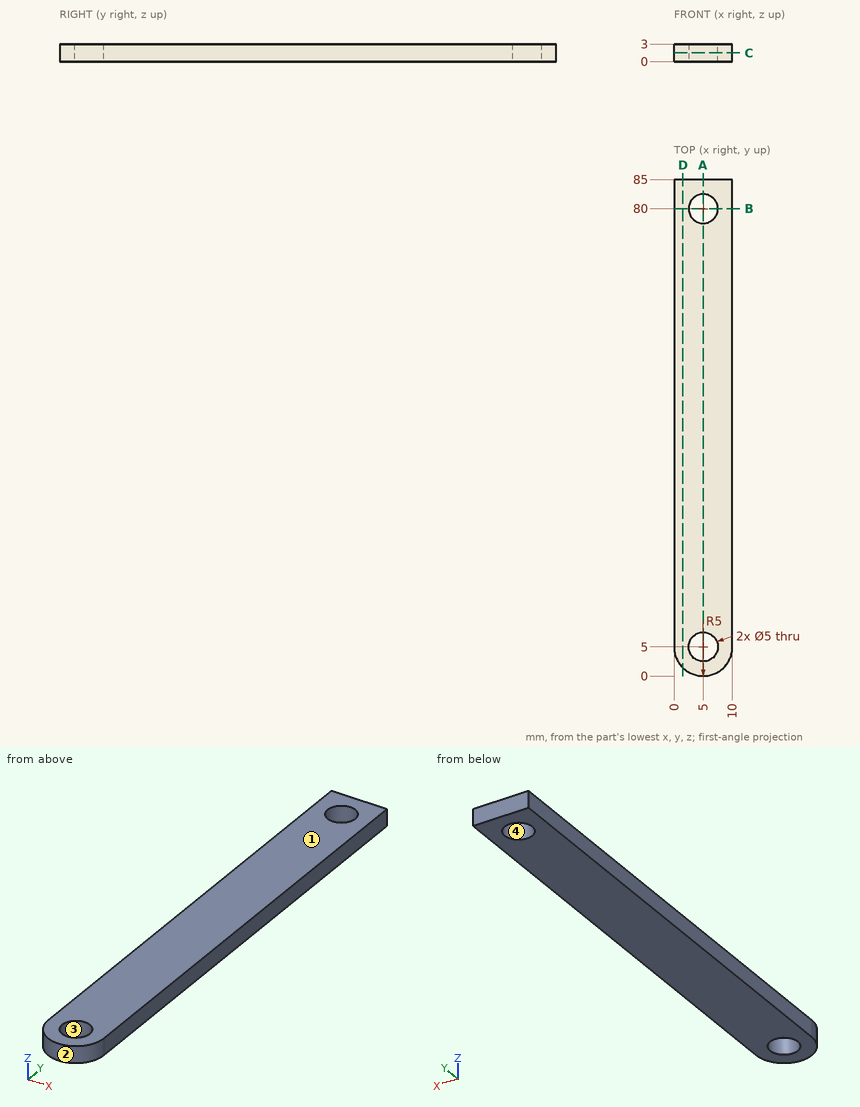
Here's the drawing with two shaded views (mm, measured from the low corner). I have some questions. Give positions to 0.01 mm unless a question says otherwise; leave off trailing zeros. Loops run counter-clockwise (first coordinate to the right, second up) from the corner with the lowest first, then second, coordinate; pieces in that order, holes last. Notation, with made-up numbers: (58.5, 62) - (99.5, 62) arc R12 cw to (99.5, 78) - close; hole circle Ø1 at (85, 56.25). An arc over 180 degrees is marked (long way). Answer in a Markdown table with one row per item. Add a question column.
Q1. We'd pull the mould along X, two halves only. Please class the marked faces 1, 2, 3 and 4: +X half, -X half, draft (parallel to the pull), parting line (faces both ways), or undercut.
Q2. If we section it at C-C (z = 1.5): List the corners of the cut face in (x, y) for me, plus the area to 3 significant figures.
Q3. If we section it at A-A (x = 5): List the corners of the cut face in (y, z) for me, plus the area to 3 significant figures.
Q4. If we section it at B-B (y = 80): List the corners of the cut face in (x, z) for me.
Q5. If we section it at D-D (x = 1.5): List the corners of the cut face in (y, z) for me.
Q6. Please list where these lines run through material, in increasing order: L1, parallel to Y at x = 5, z = 1.4; L2, parallel to X at y = 80, z = 2.05; L3, parallel to Y at x = 4, z = 0.65. Write a range as from..to.
The answers:
| question | item | result |
|---|---|---|
| 1 | face 1 | draft |
| 1 | face 2 | parting line |
| 1 | face 3 | undercut |
| 1 | face 4 | undercut |
| 2 | outline | (0, 5) arc R5 ccw to (10, 5) - (10, 85) - (0, 85) - close; hole circle Ø5 at (5, 5); hole circle Ø5 at (5, 80) |
| 2 | area | 800 mm^2 |
| 3 | outline | (0, 0) - (2.5, 0) - (2.5, 3) - (0, 3) - close; (7.5, 0) - (77.5, 0) - (77.5, 3) - (7.5, 3) - close; (82.5, 0) - (85, 0) - (85, 3) - (82.5, 3) - close |
| 3 | area | 225 mm^2 |
| 4 | outline | (0, 0) - (2.5, 0) - (2.5, 3) - (0, 3) - close; (7.5, 0) - (10, 0) - (10, 3) - (7.5, 3) - close |
| 5 | outline | (1.43, 0) - (85, 0) - (85, 3) - (1.43, 3) - close |
| 6 | L1 | y = 0..2.5, 7.5..77.5, 82.5..85 |
| 6 | L2 | x = 0..2.5, 7.5..10 |
| 6 | L3 | y = 0.1..2.71, 7.29..77.71, 82.29..85 |
